from build123d import *

# Parameters (mm, degrees)
SKETCH1_W           = 25
SKETCH1_H           = 40.5
BOSS_EXTRUDE1_DEPTH = 2
SKETCH2_W           = 25
SKETCH2_H           = 20
BOSS_EXTRUDE2_DEPTH = 2
SKETCH3_W           = 25
SKETCH3_H           = 20
BOSS_EXTRUDE3_DEPTH = 2
SKETCH5_R           = 4
CUT_EXTRUDE2_DEPTH  = 21
SKETCH6_R           = 1.5
CUT_EXTRUDE3_DEPTH  = 21
SKETCH7_R           = 1
CUT_EXTRUDE4_DEPTH  = 55


with BuildPart() as part:
    # Sketch1 → Boss-Extrude1 (new body)
    with BuildSketch(Plane.XY):
        with Locations((-0.174770451, 10.252942624)):
            Rectangle(SKETCH1_W, SKETCH1_H)
    extrude(amount=BOSS_EXTRUDE1_DEPTH)

    # Sketch2 → Boss-Extrude2 (add)
    with BuildSketch(Plane(origin=(0, 30.502942624, 0), x_dir=(1, 0, 0), z_dir=(0, 1, 0))):
        with Locations((-0.174770451, -10)):
            Rectangle(SKETCH2_W, SKETCH2_H)
    extrude(amount=BOSS_EXTRUDE2_DEPTH)

    # Sketch3 → Boss-Extrude3 (add)
    with BuildSketch(Plane(origin=(0, -9.997057376, 0), x_dir=(-1, 0, 0), z_dir=(0, -1, 0))):
        with Locations((0.174770451, -10)):
            Rectangle(SKETCH3_W, SKETCH3_H)
    extrude(amount=BOSS_EXTRUDE3_DEPTH)

    # Sketch5 → Cut-Extrude2 (cut)
    with BuildSketch(Plane(origin=(0, 0, 0), x_dir=(-1, 0, 0), z_dir=(0, 0, -1))):
        with Locations((0.174770451, 10.252942624)):
            Circle(SKETCH5_R)
    extrude(amount=-CUT_EXTRUDE2_DEPTH, mode=Mode.SUBTRACT)

    # Sketch6 → Cut-Extrude3 (cut)
    with BuildSketch(Plane(origin=(0, 0, 0), x_dir=(-1, 0, 0), z_dir=(0, 0, -1))):
        with Locations((7.174770451, 10.252942624)):
            Circle(SKETCH6_R)
        with Locations((0.174770451, 3.252942624)):
            Circle(SKETCH6_R)
        with Locations((-6.825229549, 10.252942624)):
            Circle(SKETCH6_R)
        with Locations((0.174770451, 17.252942624)):
            Circle(SKETCH6_R)
    extrude(amount=-CUT_EXTRUDE3_DEPTH, mode=Mode.SUBTRACT)

    # Sketch7 → Cut-Extrude4 (cut)
    with BuildSketch(Plane(origin=(0, -11.997057376, 0), x_dir=(-1, 0, 0), z_dir=(0, -1, 0))):
        with Locations(Location((7.174770451, -15.473202344, 0), (0, 0, 90))):
            Circle(SKETCH7_R)
        with Locations(Location((-6.817230105, -15, 0), (0, 0, 90))):
            Circle(SKETCH7_R)
        with Locations(Location((0.174770451, -8, 0), (0, 0, 90))):
            Circle(SKETCH7_R)
    extrude(amount=-CUT_EXTRUDE4_DEPTH, mode=Mode.SUBTRACT)


solid = part.part
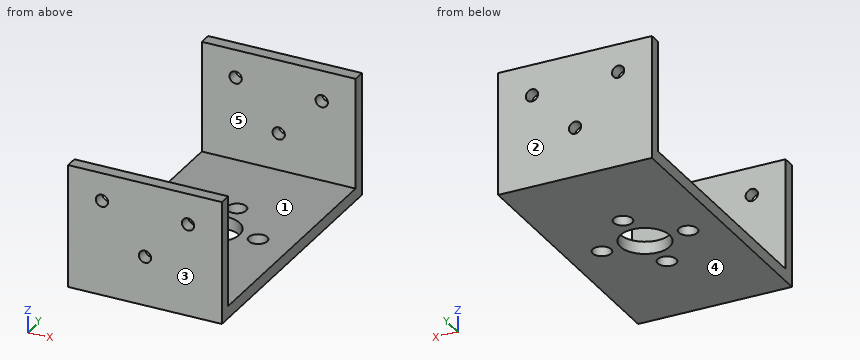
CAD build for the part. Positions are in the model's coordinates, mm. Face numbers are marked on the shaded views. A direction names the side the tool comes from. Give positions to 0.01 mm unless a question says otherwise; leave off trailing zeros. Order: outer loops, then holes, each group sorted by start corner. A loop starts at its lowest first (then second) coordinate and runs counter-clockwise, first axis right, second up. Notation, with made-up numbers: (-36, 26) -> (16, 26) arc R24 ccw to (16, 40) -> close; hole circle Ø5 at (-2, 13.25). An arc over 180 degrees is marked (long way). Return JSON: item names as keys, results as strings.
Q1. Which spindle directions (+Z, -Z, +X, -X, +Y, -Y) get a long thin tool onto all of the face, cutting with end or side? Do the marked faces 1 and 2. Say none if no direction does.
Working result:
{"face 1": "+Z, +X, -X", "face 2": "+Z, -Z, +X, -X, +Y"}
Q2. Drill centre lines: line 1 (Y direction, x = 7.75, z = 13.25); line 2 (Z direction, x = 6.25, y = 18); line 3 (X direction, y = -11.1, z = 15). Where is each one in solid material? Low to high.
Working result:
{"line 1": "-12 to -10, 30.5 to 32.5", "line 2": "0 to 2", "line 3": "-12.67 to -8.06, -6.29 to 5.82, 7.82 to 12.33"}
Q3. Saw through at B-B (z = 18.25). Write the cut outline in (x, y), then the cut area to 3 significant figures.
Working result:
{"outline": "(-12.67, -12) -> (12.33, -12) -> (12.33, -10) -> (-12.67, -10) -> close; (-12.67, 30.5) -> (12.33, 30.5) -> (12.33, 32.5) -> (-12.67, 32.5) -> close", "area": "100 mm²"}
Q4. Saw through at C-C (z = 15). Write the cut outline in (x, y).
Working result:
{"outline": "(-12.67, -12) -> (-8.06, -12) -> (-8.06, -10) -> (-12.67, -10) -> close; (-12.67, 30.5) -> (-8.06, 30.5) -> (-8.06, 32.5) -> (-12.67, 32.5) -> close; (-6.29, -12) -> (5.82, -12) -> (5.82, -10) -> (-6.29, -10) -> close; (-6.29, 30.5) -> (5.82, 30.5) -> (5.82, 32.5) -> (-6.29, 32.5) -> close; (7.82, -12) -> (12.33, -12) -> (12.33, -10) -> (7.82, -10) -> close; (7.82, 30.5) -> (12.33, 30.5) -> (12.33, 32.5) -> (7.82, 32.5) -> close"}
Q5. Mould opens along Y. For the marked faces 3, 4 and 5 say: pulls with the +Y half, pulls with the -Y half, needs draft (parallel to the pull), parting line crosses it, or undercut.
Working result:
{"face 3": "pulls with the -Y half", "face 4": "needs draft", "face 5": "undercut"}
Q6. Flat gauge pin, fed straight in: pin 1 (7.5 mm diameter, centred on x = 5, y = 4, fed in from +Z). Where does the tip first touch, or does it go through?
Working result:
{"pin 1": "z = 2"}
Q7. Saw through at D-D (y = 15). Write the cut outline in (x, z), then the cut area to 3 significant figures.
Working result:
{"outline": "(-12.67, 0) -> (12.33, 0) -> (12.33, 2) -> (-12.67, 2) -> close", "area": "50.0 mm²"}
Q8. Saw through at A-A (z = 8). Write the cut outline in (x, y).
Working result:
{"outline": "(-12.67, -12) -> (-1.17, -12) -> (-1.17, -10) -> (-12.67, -10) -> close; (-12.67, 30.5) -> (-1.17, 30.5) -> (-1.17, 32.5) -> (-12.67, 32.5) -> close; (0.83, -12) -> (12.33, -12) -> (12.33, -10) -> (0.83, -10) -> close; (0.83, 30.5) -> (12.33, 30.5) -> (12.33, 32.5) -> (0.83, 32.5) -> close"}
